For this review, take the finished solid that the model builds, in its own axes (mm). A direction names the side the tool comes from. Coordinates: 2 decimals unless noted, no trailing zeros. Loops run counter-clockwise (first coordinate to the right, second up) from the corner with the lowest first, then second, coordinate; pieces in that order, holes last. Notation, with made-up numbers: (88, -22) - (118, -22) arc R25 ccw to (118, 15) - close; hole circle Ø2 at (70, 73.25). An arc over 180 degrees is marked (long way). Use one line per item in the form item = value. Start each with the question number.
1. For pin 1 Ø5 at (y, z) = (247, 37) entering from -X; pin 2 Ø2.5 at (y, z) = (245, 35) entering from +X; pin 3 Ø8 at (x, y) = (96, 118.5) entering from +Z; pin 4 Ø4 at (x, y) = (171.5, 91) entering from +Z, all flat-tipped, find the tip position at first contact; note any pin that passes through.
2. Machinability: for faces 4 (the face through (7, 127, 8)), 5 (the face through (183, 156, 29)), 6 (the face through (50, 244.9, 32.7)), 7 (the face through (187, 250, 25)), 8 (the face through (320, 245.1, 32.7)), which of the approach directions +Z, -Z, +X, -X, +Y, -Y give a long, thin tool a straight path to every point of the face, cutting with its end or side? Answer none if there is none.
3. Add section D-D on y = 231. Give the boundary of the cut face in (x, z), and give its area (3 significant figures).
4. To check wall thickness, follow probe 1 along Z at (x, y) = (113.5, 245); probe 2 along Y at (x, z) = (283.5, 35); probe 3 along Z at (x, y) = (74.5, 134.5). State the ranges of each line that lie inside material, in increasing order.
5. Add section C-C on y = 176. Give the boundary of the cut face in (x, z), and give its area (3 significant figures).
6. Draft analysis for pull direction X (two halves, no side actions). For faces 1 (the face through (365, 5, 22)), 2 (the face through (184, 50, 29)), 3 (the face through (182, 242, 7)), state which applies: +X half, -X half, draft (parallel to the pull), parting line (faces both ways), or undercut.
7. Add section B-B on x = 35. Give the boundary of the cut face in (y, z), and give its area (4 significant figures).
Autodesk Inventor part; units mm, degrees
ref_plane "YZ Plane" through (0, 0, 0) normal (1, 0, 0) x (0, 1, 0)
ref_plane "XZ Plane" through (0, 0, 0) normal (0, 1, 0) x (-1, 0, 0)
ref_plane "XY Plane" through (0, 0, 0) normal (0, 0, 1) x (1, 0, 0)
sketch "スケッチ1" plane through (0, 0, 0) normal (0, 0, 1) x (1, 0, 0)
  line L0 (0, 0) -> (370, 0)
  line L1 (370, 0) -> (370, 250)
  line L2 (370, 250) -> (0, 250)
  line L3 (0, 250) -> (0, 0)
  dimension "d0" = 370
  dimension "d1" = 250
extrude "押し出し1" add sketch "スケッチ1" along normal blind 30
sketch "スケッチ2" plane through (0, 0, 30) normal (0, 0, 1) x (1, 0, 0)
  line L0 (370, 250) -> (0, 250)
  line L1 (50, 250) -> (320, 250)
  line L2 (320, 250) -> (320, 240)
  line L3 (320, 240) -> (50, 240)
  line L4 (50, 240) -> (50, 250)
  line L5 (0, 250) -> (0, 0)
  line L6 (370, 0) -> (370, 250)
  dimension "d4" = 50
  dimension "d5" = 50
  dimension "d6" = 10
extrude "押し出し2" add sketch "スケッチ2" along normal blind 10
fillet "フィレット1" radius 5 2 edges at (185, 240, 40) (185, 250, 40)
chamfer "面取り1" distance 15 angle 45 4 edges at (185, 0, 0) (0, 125, 0) (370, 125, 0) (185, 250, 0)
sketch "スケッチ3" plane through (0, 0, 30) normal (0, 0, 1) x (1, 0, 0)
  line L0 (0, 0) -> (370, 0)
  line L1 (185, 0) -> (185, 50) construction
  line L2 (135, 20) -> (235, 20)
  line L3 (235, 20) -> (235, 80)
  line L4 (235, 80) -> (135, 80)
  line L5 (135, 80) -> (135, 20)
  line L6 (135, 20) -> (235, 80) construction
  line L7 (235, 20) -> (135, 80) construction
  line L8 (185, 50) -> (185, 155) construction
  line L9 (30, 210) -> (340, 210)
  line L10 (340, 210) -> (340, 100)
  line L11 (340, 100) -> (30, 100)
  line L12 (30, 100) -> (30, 210)
  line L13 (30, 210) -> (340, 100) construction
  line L14 (340, 210) -> (30, 100) construction
  line L15 (370, 250) -> (320, 250) construction
  line L16 (370, 0) -> (370, 250) construction
  dimension "d13" = 60
  dimension "d14" = 100
  dimension "d15" = 20
  dimension "d16" = 20
  dimension "d17" = 40
  dimension "d18" = 30
extrude "押し出し3" cut sketch "スケッチ3" against normal blind 1
chamfer "面取り2" distance 10 angle 45 4 edges at (370, 0, 22.5) (0, 0, 22.5) (370, 250, 22.5) (0, 250, 22.5)
sketch "スケッチ4" plane through (320, 240, 30) normal (1, 0, 0) x (0, 0, -1)
  arc A0 (-5, 10) -> (-5, 0) centre (-5, 5) ccw
  circle A1 centre (-5, 5) radius 2
  point P0 (30, -240)
  dimension "d24" = 4
extrude "押し出し4" cut sketch "スケッチ4" against normal up to next
properties part number "PCパーツ1"
Conclusion:
q1.pin_1 = 50
q1.pin_2 = through
q1.pin_3 = 29
q1.pin_4 = 30
q2.face_4 = -Z, -X, +Y, -Y
q2.face_5 = +Z
q2.face_6 = +Z, -X, +Y, -Y
q2.face_7 = +Z, -Z, +X, -X, +Y
q2.face_8 = +Z, +X, +Y, -Y
q3.outline = (0, 15) - (15, 0) - (355, 0) - (370, 15) - (370, 30) - (0, 30) - close
q3.area = 10,900 mm^2
q4.probe_1 = 10 to 33, 37 to 40
q4.probe_2 = 240 to 243, 247 to 250
q4.probe_3 = 0 to 29
q5.outline = (0, 15) - (15, 0) - (355, 0) - (370, 15) - (370, 30) - (340, 30) - (340, 29) - (30, 29) - (30, 30) - (0, 30) - close
q5.area = 10,600 mm^2
q6.face_1 = +X half
q6.face_2 = undercut
q6.face_3 = draft
q7.outline = (0, 15) - (15, 0) - (235, 0) - (250, 15) - (250, 30) - (210, 30) - (210, 29) - (100, 29) - (100, 30) - (0, 30) - close
q7.area = 7,165 mm^2
